```python
from build123d import *


with BuildPart() as part:
    # Esquisse1 → Révolution1 (revolve)
    with BuildSketch(Plane.XY, mode=Mode.PRIVATE) as r_volution1_sk:
        with BuildLine():
            Line((2, 0), (4, 0))
            Line((4, 0), (4.5, -0.5))
            Line((4.5, -0.5), (4.5, -1))
            Line((4.5, -1), (4, -1.5))
            Line((4, -1.5), (3.5, -1.5))
            ThreePointArc((3.5, -1.5), (3.146446609, -1.646446609), (3, -2))
            Line((3, -2), (3, -5.5))
            Line((3, -5.5), (2.5, -6))
            Line((2.5, -6), (2, -6))
            Line((2, -6), (1.5, -5.5))
            Line((1.5, -5.5), (1.5, -0.5))
            Line((1.5, -0.5), (2, 0))
        make_face()
    revolve(r_volution1_sk.sketch.rotate(Axis((0, 0, 0), (0, -1, 0)), 90), axis=Axis((0, 0, 0), (0, -1, 0)))


solid = part.part
```
Could you check a few things on this model? Use its own coordinates, in mm. A direction names the side the tool comes from. Coordinates: 2 decimals unless noted, no trailing zeros. Write each loop counter-clockwise with the first axis right and the second up, starting at its lowest first coordinate (ties: lowest second). Pieces come first, ordered by that corner, then holes. Notation, with made-up numbers: (63, 12.5) - (122, 12.5) arc R19 cw to (122, 35.5) - close; hole circle Ø6 at (-34.75, -36.5). An arc over 180 degrees is marked (long way). Use a Markdown table: item, result.
Q1. Imagine slicing it at C-C (y = -5.2). List the corners of the cut face in (x, z) for me, and give its area (3 significant figures).
Geometry check:
| item | result |
|---|---|
| outline | circle Ø6 at (0, 0); hole circle Ø3 at (0, 0) |
| area | 21.2 mm2 |
Q2. Which directions (+Z, -Z, +X, -X, +Y, -Y) give clear straight access to the entire face, cutting with the end or side of a thin tool? Please do faces 1 (the flat face through (-2, 0, -1)), 2 (the cylindrical face through (-0.9, -3.77, 2.86)).
Geometry check:
| item | result |
|---|---|
| face 1 | +Z, -Z, +X, -X, +Y |
| face 2 | -Y |
Q3. I'm going to push flat-ended pins straight in: pin 1 Ø1 at (x, y) = (-2.5, -4.5) entering from +Z; pin 2 Ø4 at (x, z) = (2, 2) entering from +Y. Where does each tip first touch, or does it pass through?
Geometry check:
| item | result |
|---|---|
| pin 1 | stops at z = 2.24 |
| pin 2 | stops at y = 0 |
Q4. Please list where these lines run through material, in increasing order: L1, parallel to X at y = -2.65, z = 0; L2, parallel to Y at x = 3.5, z = 0.25; L3, parallel to Z at x = 1, y = -2.8.
Geometry check:
| item | result |
|---|---|
| L1 | x = -3 to -1.5, 1.5 to 3 |
| L2 | y = -1.5 to 0 |
| L3 | z = -2.83 to -1.12, 1.12 to 2.83 |
Q5. Imagine slicing it at B-B (z = 0). List the corners of the cut face in (x, y) for me, and give its area (3 significant figures).
Geometry check:
| item | result |
|---|---|
| outline | (-4.5, -1) - (-4, -1.5) - (-3.5, -1.5) arc R0.5 cw to (-3, -2) - (-3, -5.5) - (-2.5, -6) - (-2, -6) - (-1.5, -5.5) - (-1.5, -0.5) - (-2, 0) - (-4, 0) - (-4.5, -0.5) - close; (1.5, -5.5) - (2, -6) - (2.5, -6) - (3, -5.5) - (3, -2) arc R0.5 cw to (3.5, -1.5) - (4, -1.5) - (4.5, -1) - (4.5, -0.5) - (4, 0) - (2, 0) - (1.5, -0.5) - close |
| area | 21.4 mm2 |
Q6. Thinking about a two-plate mould opening in X: for faces 3 (the cylindrical face through (-0.45, -2.96, 1.43)), 4 (the flat face through (-2, -6, -1)), 5 (the cylindrical face through (-3.04, -0.75, -3.32)), which applies, +X half, -X half, draft (parallel to the pull), parting line (faces both ways), or undercut?
Geometry check:
| item | result |
|---|---|
| face 3 | undercut |
| face 4 | draft |
| face 5 | parting line |
Q7. Imagine slicing it at A-A (x = 0). List the corners of the cut face in (y, z) for me.
Geometry check:
| item | result |
|---|---|
| outline | (-6, -2.5) - (-5.5, -3) - (-2, -3) arc R0.5 cw to (-1.5, -3.5) - (-1.5, -4) - (-1, -4.5) - (-0.5, -4.5) - (0, -4) - (0, -2) - (-0.5, -1.5) - (-5.5, -1.5) - (-6, -2) - close; (-6, 2) - (-5.5, 1.5) - (-0.5, 1.5) - (0, 2) - (0, 4) - (-0.5, 4.5) - (-1, 4.5) - (-1.5, 4) - (-1.5, 3.5) arc R0.5 cw to (-2, 3) - (-5.5, 3) - (-6, 2.5) - close |
